Part model, mm, in its own coordinate system. Round coordinates to 2 decimals unless told otherwise and drop trailing zeros. Write each loop counter-clockwise with the first axis right and the second up, starting at its lowest first coordinate (ties: lowest second). Pieces come first, ordered by that corner, then holes.
```python
from build123d import *

# Parameters (mm, degrees)
F2_R     = 5
F6_DEPTH = 35


with BuildPart() as f3:
    # F3: sweep along a path in F0
    with BuildLine(Plane.XY) as f3_path:
        Line((-5.5, 90), (-5.5, 39.1120186132))
        ThreePointArc((-5.5, 39.1120186132), (-7.9944448559, 25.2075828701), (-15.1666666667, 13.0373395377))
        ThreePointArc((-15.1666666667, 13.0373395377), (0, -20), (15.1666666667, 13.0373395377))
        ThreePointArc((15.1666666667, 13.0373395377), (7.9944448559, 25.2075828701), (5.5, 39.1120186132))
        Line((5.5, 39.1120186132), (5.5, 2000))
    # F2 (on plane+point) → F3 (sweep)
    with BuildSketch(Plane.XZ.offset(-90)):
        with Locations((-5.5, 0)):
            Circle(F2_R)
    sweep(path=f3_path.line)

    # F5 (on offset) → F6 (join)
    with BuildSketch(Plane.XZ.offset(-80)):
        with BuildLine():
            Line((-5.5, -10.0000000344), (5.5, -10.0000000344))
            ThreePointArc((5.5, -10.0000000344), (15.5000000344, 0), (5.5, 10.0000000344))
            Line((5.5, 10.0000000344), (-5.5, 10.0000000344))
            ThreePointArc((-5.5, 10.0000000344), (-15.5000000344, 0), (-5.5, -10.0000000344))
        make_face()
        with BuildLine():
            ThreePointArc((-5.5, -5), (-10.5, 0), (-5.5, 5))
            Line((-5.5, 5), (5.5, 5))
            ThreePointArc((5.5, 5), (10.5, 0), (5.5, -5))
            Line((5.5, -5), (-5.5, -5))
        make_face(mode=Mode.SUBTRACT)
    extrude(amount=F6_DEPTH)


solid = f3.part
```
Q1. Cut at B-B on y = 1540. Write the cut outline in (x, z).
Values follow:
outline: circle Ø10 at (5.5, 0)
Q2. Wall check: L1, parallel to Z at x = 7, y = 1761.5; L2, parallel to X at y = 1717, z = 0; L3, parallel to Y at x = 5, z = 7.75. Give the ranges that are in metal, low to high.
Values follow:
L1: z = -4.77 to 4.77
L2: x = 0.5 to 10.5
L3: y = 45 to 80
Q3. Cut at A-A on z = 0. Write the cut outline in (x, y) (3 decimals), plus the area to 3 significant figures.
Values follow:
outline: (-18.958, 16.297) arc R25 ccw (long way) to (18.958, 16.297) arc R35 cw to (10.5, 39.112) - (10.5, 45) - (15.5, 45) - (15.5, 80) - (10.5, 80) - (10.5, 2000) - (0.5, 2000) - (0.5, 39.112) arc R45 ccw to (11.375, 9.778) arc R15 cw (long way) to (-11.375, 9.778) arc R45 ccw to (-0.5, 39.112) - (-0.5, 90) - (-10.5, 90) - (-10.5, 80) - (-15.5, 80) - (-15.5, 45) - (-10.5, 45) - (-10.5, 39.112) arc R35 cw to start
area: 21,900 mm2
Q4. Drop flat-ended pins along their axis: pin 1 (12 mm diameter, centred on y = 491, z = -7, fed in from -X); pin 2 (5 mm diameter, centred on y = 828.5, z = 5, fed in from +X); pin 3 (12 mm diameter, centred on y = 1271, z = 0, fed in from -X). Give the stop position or say it passes through.
Values follow:
pin 1: stops at x = 0.6
pin 2: stops at x = 9.83
pin 3: stops at x = 0.5
